Here's the drawing with two shaded views (mm, measured from the low corner). I have some questions. A direction names the side the tool comes from. Coordinates: 2 decimals unless noted, no trailing zeros. Write each loop counter-clockwise with the first axis right and the second up, starting at its lowest first coordinate (ties: lowest second). Pieces come first, ordered by that corner, then holes.
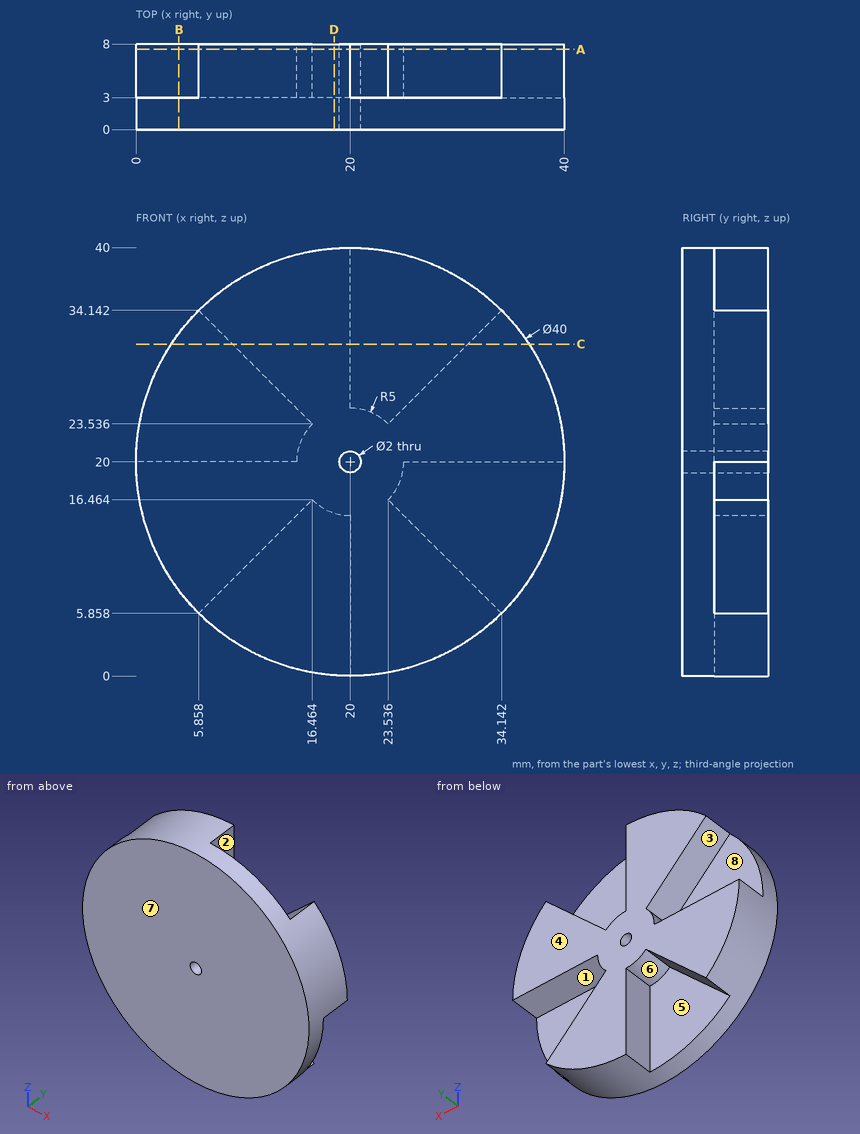
1. If we mould it in two halves opening along Z, with no side actions, what happens to the marked faces 6, 7 and 8? For each: pulls with the +Z half, pulls with the -Z half, needs draft (parallel to the pull), parting line crosses it, or undercut.
Verdict:
face 6: pulls with the -Z half
face 7: needs draft
face 8: undercut
2. For pin 1 (4 mm diameter, centred on y = 2.5, z = 11, fed in from -X) (1 decimal); pin 2 (4 mm diameter, centred on x = 9, y = 6, fed in from +Z); pin 3 (4 mm diameter, centred on y = 4.5, z = 6.5, fed in from -X), each with a flat end and sliding along its axis, tell me the tip position at first contact or that it passes through.
Verdict:
pin 1: stops at x = 1.3
pin 2: stops at z = 37.86
pin 3: stops at x = 3.64
3. On a 3-axis mill with a long thin cutter (end or side, diameter ignored), from which of +Z, -Z, +X, -X, +Y, -Y can I reach the whole of each face in a straight line? I mean the marked faces 1, 2, 3, 4 and 5. Say none if no direction works.
Verdict:
face 1: +X, +Y
face 2: +Z, +Y
face 3: -X, +Y
face 4: +Z, -Z, +X, -X, +Y
face 5: -Z, +Y
4. Please list where these lines run through material, in increasing order: line 1 along X through (y, z) = (2.75, 20); line 2 along Y through (x, z) = (5.5, 32); line 3 along Z through (x, y) = (14.5, 7.5).
Verdict:
line 1: x = 0 to 19, 21 to 40
line 2: y = 0 to 3
line 3: z = 14.5 to 20, 25.5 to 39.23
5. I want a section at B-B on x = 4. Please give me the cut outline in (y, z), plus the area to 3 significant figures.
Verdict:
outline: (0, 8) - (8, 8) - (8, 20) - (3, 20) - (3, 32) - (0, 32) - close
area: 132 mm2
6. I want a section at C-C on z = 31. Please give me the cut outline in (x, y).
Verdict:
outline: (3.3, 0) - (36.7, 0) - (36.7, 8) - (31, 8) - (31, 3) - (20, 3) - (20, 8) - (9, 8) - (9, 3) - (3.3, 3) - close
7. I want a section at D-D on x = 18.5. Please give me the cut outline in (y, z).
Verdict:
outline: (0, 0.06) - (3, 0.06) - (3, 15.23) - (8, 15.23) - (8, 39.94) - (0, 39.94) - close
8. I want a section at A-A on y = 7.5. Please give me the cut outline in (x, z) (1 decimal).
Verdict:
outline: (0, 20) arc R20 ccw to (5.9, 5.9) - (16.5, 16.5) arc R5 ccw to (20, 15) - (20, 0) arc R20 ccw to (34.1, 5.9) - (23.5, 16.5) arc R5 ccw to (25, 20) - (40, 20) arc R20 ccw to (34.1, 34.1) - (23.5, 23.5) arc R5 ccw to (20, 25) - (20, 40) arc R20 ccw to (5.9, 34.1) - (16.5, 23.5) arc R5 ccw to (15, 20) - close; hole circle Ø2 at (20, 20)
